Source: CAD feature listing. Evaluate the final solid. Frame: model axes, mm. Face numbers are marked on the shaded views. A direction names the side the tool comes from. Round coordinates to 2 decimals unless told otherwise and drop trailing zeros. Write each loop counter-clockwise with the first axis right and the second up, starting at its lowest first coordinate (ties: lowest second). Pieces come first, ordered by that corner, then holes.
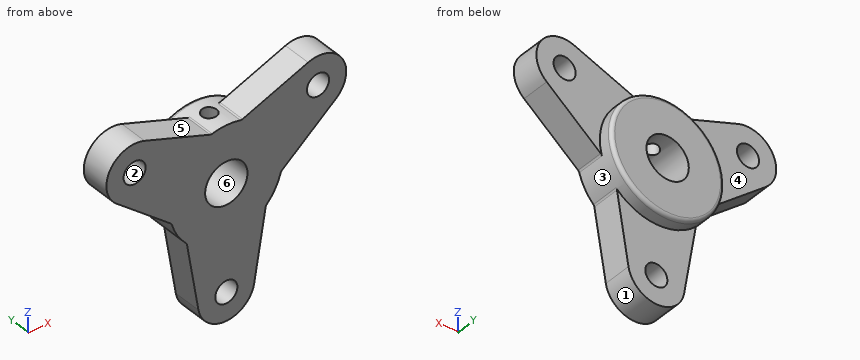
from build123d import *

# Parameters (mm, degrees)
SKETCH1_R                        = 12.7
SKETCH1_R_2                      = 4.7625
BOSS_EXTRUDE1_DEPTH              = 6.35
BOSS_EXTRUDE2_START              = 3.175
SKETCH1_5_R                      = 12.7
SKETCH1_5_R_2                    = 4.7625
BOSS_EXTRUDE2_DEPTH              = 3.175
F_10_CLEARANCE_HOLE1_D           = 4.9784
TAP_DRILL_FOR_M4X0_7_TAP1_REACH  = 52.866
TAP_DRILL_FOR_M4X0_7_TAP1_BORE_R = 1.65
FILLET1_R                        = 0.79375


with BuildPart() as part:
    # Sketch1 → Boss-Extrude1 (new body)
    # profile 1 of 4: a face of its own
    with BuildSketch(Plane(origin=(0, 0, 0), x_dir=(1, 0, 0), z_dir=(0, 1, 0))):
        with BuildLine():
            ThreePointArc((6.263906023, 24.854604283), (0, 30.1625), (-6.263906023, 24.854604283))
            Line((-6.263906023, 24.854604283), (-8.89, 9.069614104))
            ThreePointArc((-8.89, 9.069614104), (0, 12.7), (8.89, 9.069614104))
            Line((8.89, 9.069614104), (6.263906023, 24.854604283))
        make_face()
    # profile 2 of 4: a face of its own
    with BuildSketch(Plane(origin=(0, 0, 0), x_dir=(1, 0, 0), z_dir=(0, 1, 0))):
        Circle(SKETCH1_R)
        with Locations(Location((0, 0, 0), (0, 0, 270))):
            Circle(SKETCH1_R_2, mode=Mode.SUBTRACT)
    # profile 3 of 4: a face of its own
    with BuildSketch(Plane(origin=(0, 0, 0), x_dir=(1, 0, 0), z_dir=(0, 1, 0))):
        with BuildLine():
            Line((24.656671722, -7.002600399), (12.299516217, 3.164158788))
            ThreePointArc((12.299516217, 3.164158788), (12.599481258, 1.594701233), (12.7, 0))
            ThreePointArc((12.7, 0), (10.114120228, -7.680792409), (3.409516217, -12.233772892))
            Line((3.409516217, -12.233772892), (18.392765699, -17.852003884))
            ThreePointArc((18.392765699, -17.852003884), (26.121491242, -15.08125), (24.656671722, -7.002600399))
        make_face()
    # profile 4 of 4: a face of its own
    with BuildSketch(Plane(origin=(0, 0, 0), x_dir=(1, 0, 0), z_dir=(0, 1, 0))):
        with BuildLine():
            ThreePointArc((-3.409516217, -12.233772892), (-10.998522628, -6.35), (-12.299516217, 3.164158788))
            Line((-12.299516217, 3.164158788), (-24.656671722, -7.002600399))
            ThreePointArc((-24.656671722, -7.002600399), (-26.121491242, -15.08125), (-18.392765699, -17.852003884))
            Line((-18.392765699, -17.852003884), (-3.409516217, -12.233772892))
        make_face()
    extrude(amount=-BOSS_EXTRUDE1_DEPTH)

    # Sketch1<5> → Boss-Extrude2 (add)
    with BuildSketch(Plane(origin=(0, 0, 0), x_dir=(1, 0, 0), z_dir=(0, 1, 0)).offset(BOSS_EXTRUDE2_START)):
        with Locations(Location((0, 0, 0), (0, 0, 270))):
            Circle(SKETCH1_5_R)
        with Locations(Location((0, 0, 0), (0, 0, 270))):
            Circle(SKETCH1_5_R_2, mode=Mode.SUBTRACT)
    extrude(amount=-BOSS_EXTRUDE2_DEPTH)

    # #10 Clearance Hole1 (through all)
    with Locations(Plane(origin=(0, 0, -23.8125), x_dir=(0, 0, 1), z_dir=(0, 1, 0))):
        with Locations((0, 0), (35.71875, 20.622229928), (35.71875, -20.622229928)):
            Hole(F_10_CLEARANCE_HOLE1_D / 2)

    # Tap Drill for M4x0.7 Tap1 bore (on position points) → Tap Drill for M4x0.7 Tap1 (cut, up to next)
    with BuildSketch(Plane(origin=(0, -1.5875, 12.7), x_dir=(1, 0, 0), z_dir=(0, 0, 1)), mode=Mode.PRIVATE) as tap_drill_for_m4x0_7_tap1_sk1:
        Circle(TAP_DRILL_FOR_M4X0_7_TAP1_BORE_R)
    tap_drill_for_m4x0_7_tap1_tool1 = extrude(tap_drill_for_m4x0_7_tap1_sk1.sketch, amount=-TAP_DRILL_FOR_M4X0_7_TAP1_REACH, mode=Mode.PRIVATE) & part.part
    add(tap_drill_for_m4x0_7_tap1_tool1.solids().sort_by_distance((0, -1.5875, 12.7))[0], mode=Mode.SUBTRACT)

    # Fillet1
    # the kernel refuses this fillet: 0.79375 mm, written as the material it adds along each edge
    with BuildSketch(Plane(origin=(8.89, 0, -9.069614104), x_dir=(0.7073032764952122, 0, 0.7069102312593428), z_dir=(0, -1, 0)), Plane(origin=(3.409516217, 0, 12.233772892), x_dir=(-0.9658538567133282, 0, 0.2590874899951552), z_dir=(0, -1, 0)), Plane(origin=(-12.299516217, 0, -3.164158788), x_dir=(0.2585505802181169, 0, -0.965997721254494), z_dir=(0, -1, 0))) as fillet1_piece_1:
        with BuildLine():
            CenterArc((0.254671056, -0.793712483), FILLET1_R, 90.557072072, 35.013262483)
            Line((-0.207054828, -0.148074604), (0, 0))
            ThreePointArc((0, 0), (0.123476876, -0.000600272), (0.246953752, 0))
        make_face()
    extrude(amount=6.35)
    with BuildSketch(Plane(origin=(12.299516217, 0, -3.164158788), x_dir=(-0.2585505802181021, 0, -0.9659977212544979), z_dir=(0, -1, 0)), Plane(origin=(-3.409516217, 0, 12.233772892), x_dir=(0.9658538567133268, 0, 0.2590874899951606), z_dir=(0, -1, 0)), Plane(origin=(-8.89, 0, -9.069614104), x_dir=(-0.7073032764952193, 0, 0.7069102312593356), z_dir=(0, -1, 0))) as fillet1_piece_2:
        with BuildLine():
            CenterArc((0.254671056, 0.793712483), FILLET1_R, 234.429665445, 35.013262483)
            Line((-0.207054828, 0.148074604), (0, 0))
            ThreePointArc((0, 0), (0.123476876, 0.000600272), (0.246953752, 0))
        make_face()
    extrude(amount=6.35)
    # the kernel refuses this fillet: 0.79375 mm, written as the material it takes off along each edge
    with BuildSketch(Plane(origin=(0, 3.175, 0), x_dir=(0, 0, 1), z_dir=(-1, 0, 0))) as fillet1_2_piece_1:
        with BuildLine():
            CenterArc((12.7 - FILLET1_R, -FILLET1_R), FILLET1_R, 0, 90)
            Line((12.7, -FILLET1_R), (12.7, 0))
            Line((12.7, 0), (12.7 - FILLET1_R, 0))
        make_face()
    revolve(axis=Axis((0, 3.175, 0), (0, 1, 0)), mode=Mode.SUBTRACT)


solid = part.part
1) Reachability of the marked faces 5 and 6 from +Z, -Z, +X, -X, +Y, -Y: full face, straight path, thin tool, end or side. Return the list, or none.
Taken from the geometry:
face 5: +Z, +Y, -Y
face 6: +Y, -Y
2) Contact query for flat-ended pins moving along their axis: P1, Ø3, axis at y = 2, z = -4, coming from the +X side; P2, Ø6.5, axis at x = -17.5, z = 11, coming from the +Y side; P3, Ø1.5, axis at y = 0.5, z = 8.5, coming from the -X side. Output: stop coordinate, or through.
Taken from the geometry:
P1: stops at x = 12.45
P2: stops at y = 0
P3: stops at x = -26.3
3) Section query B-B on x = 20. Return the cut outline in (y, z).
Taken from the geometry:
outline: (-6.35, 3.17) - (0, 3.17) - (0, 9.5) - (-6.35, 9.5) - close; (-6.35, 14.32) - (0, 14.32) - (0, 18.23) - (-6.35, 18.23) - close
4) Section query D-D on x = 13.5. Return the cut outline in (y, z).
Taken from the geometry:
outline: (-6.35, -2.18) - (0, -2.18) - (0, 16.02) - (-6.35, 16.02) - close
5) Material intervals for line 1 (Y direction, x = -13, z = 10.5); line 2 (X direction, y = -4, z = -24); line 3 (Z direction, x = -22.5, y = -2.5), sorted ascending.
Taken from the geometry:
line 1: y = -6.35 to 0
line 2: x = -6.41 to -2.48, 2.48 to 6.41
line 3: z = 5.23 to 10.27, 13.54 to 17.97
6) Pull-direction query (Z, two-part tool) for the marked faces 1, 2, 3 and 4; classes: released by +Z, released by -Z, zero draft, split by the parting line, or undercut.
Taken from the geometry:
face 1: released by -Z
face 2: undercut
face 3: split by the parting line
face 4: zero draft
7) Section query C-C on y = -0.75. State how many separate pieces and enclosed holes the cut face has, then the cut area to 3 significant figures.
Taken from the geometry:
separate pieces: 1
enclosed holes: 3
area: 1,090 mm2
